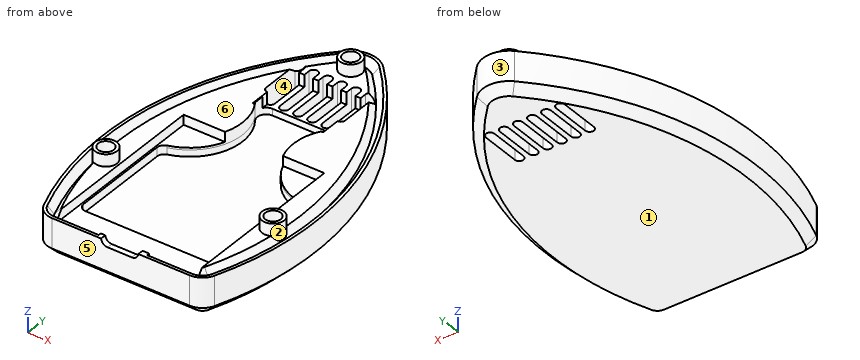
from build123d import *

# Parameters (mm, degrees)
PAD011_DEPTH           = 6.5
CHAMFER_SIZE           = 2
SKETCH020_W            = 32
SKETCH020_H            = 40
POCKET004_DEPTH        = 4.5
SKETCH021_W            = 16
SKETCH021_H            = 13
POCKET005_DEPTH        = 3
POCKET006_DEPTH        = 2
PAD012_DEPTH           = 2.5
POCKET007_DEPTH        = 5
POCKET008_DEPTH        = 6.501
LINEARPATTERN001_COUNT = 6
LINEARPATTERN001_PITCH = 2.8
POCKET009_DEPTH        = 6.501
POCKET009_DEPTH_BACK   = 6.501
LINEARPATTERN002_COUNT = 6
LINEARPATTERN002_PITCH = 3.2
SKETCH043_W            = 50
SKETCH043_H            = 9.25
PAD015_DEPTH           = 80
POCKET010_DEPTH        = 2.751
SKETCH044_R            = 2.5
PAD016_DEPTH           = 5


with BuildPart() as housing:
    # Sketch019 → Pad011 (new body, symmetric)
    with BuildSketch(Plane.XY):
        with BuildLine():
            ThreePointArc((4.279646, 74.20531), (0, 76), (-4.279646, 74.20531))
            ThreePointArc((-4.279646, 74.20531), (-22.568944, 39.95714), (-19.396798, 1.261235))
            ThreePointArc((-19.396798, 1.261235), (-17.9278, -0.59811), (-15.664513, -1.3))
            Line((15.664513, -1.3), (-15.664513, -1.3))
            ThreePointArc((15.664513, -1.3), (17.927792, -0.598116), (19.396791, 1.261217))
            ThreePointArc((19.396791, 1.261217), (22.568946, 39.95713), (4.279646, 74.20531))
        make_face()
    extrude(amount=PAD011_DEPTH, both=True)

    # Chamfer
    chamfer_edges = [housing.edges().sort_by_distance(p)[0] for p in [
        (0, -1.3, 6.5),
        (0, -1.3, -6.5),
    ]]
    chamfer(chamfer_edges, length=CHAMFER_SIZE)

    # Sketch020 → Pocket004 (cut)
    with BuildSketch(Plane.XY):
        with Locations((0, 20)):
            Rectangle(SKETCH020_W, SKETCH020_H)
    extrude(amount=POCKET004_DEPTH, mode=Mode.SUBTRACT)

    # Sketch021 → Pocket005 (cut)
    with BuildSketch(Plane.XY):
        with Locations((0, 57)):
            Rectangle(SKETCH021_W, SKETCH021_H)
    extrude(amount=POCKET005_DEPTH, mode=Mode.SUBTRACT)

    # Sketch022 → Pocket006 (cut, symmetric)
    with BuildSketch(Plane.XY):
        with BuildLine():
            ThreePointArc((-6.35, 54.4), (-8.125922, 53.319838), (-7.98356, 51.246101))
            ThreePointArc((-14.445285, 32.796789), (-6.459474, 40.356063), (-7.98356, 51.246101))
            ThreePointArc((-14.445285, 32.796789), (-15.279151, 32.221131), (-15.6, 31.26))
            Line((-15.6, 8.4), (-15.6, 31.26))
            ThreePointArc((-15.6, 8.4), (-15.131371, 7.268629), (-14, 6.8))
            Line((14, 6.8), (-14, 6.8))
            ThreePointArc((14, 6.8), (15.131371, 7.268629), (15.6, 8.4))
            Line((15.6, 31.26), (15.6, 8.4))
            ThreePointArc((15.6, 31.26), (15.279151, 32.221131), (14.445285, 32.796789))
            ThreePointArc((7.98356, 51.246101), (6.459474, 40.356063), (14.445285, 32.796789))
            ThreePointArc((7.98356, 51.246101), (8.125922, 53.319838), (6.35, 54.4))
            Line((6.35, 54.4), (-6.35, 54.4))
        make_face()
    extrude(amount=POCKET006_DEPTH, both=True, mode=Mode.SUBTRACT)

    # Sketch039 → Pad012 (join)
    with BuildSketch(Plane.XY.offset(-0.5)):
        with BuildLine():
            ThreePointArc((-4.584919, 45.32271), (-5.584919, 44.32271), (-4.584919, 43.32271))
            Line((-4.584919, 43.32271), (4.584919, 43.32271))
            ThreePointArc((4.584919, 43.32271), (5.584919, 44.32271), (4.584919, 45.32271))
            Line((4.584919, 45.32271), (-4.584919, 45.32271))
        make_face()
    extrude(amount=PAD012_DEPTH)

    # Sketch023 → Pocket007 (cut, symmetric)
    with BuildSketch(Plane.XZ):
        with BuildLine():
            ThreePointArc((-3, 3.9), (-4.5, 2.4), (-3, 0.9))
            Line((-3, 0.9), (2.5, 0.9))
            ThreePointArc((2.5, 0.9), (4, 2.4), (2.5, 3.9))
            Line((2.5, 3.9), (-3, 3.9))
        make_face()
    extrude(amount=POCKET007_DEPTH, both=True, mode=Mode.SUBTRACT)

    # Sketch025 → Pocket008 (cut, through all)
    with BuildSketch(Plane.XY):
        with BuildLine():
            ThreePointArc((-6.25, 32.5), (-7, 33.25), (-7.75, 32.5))
            Line((-7.75, 32.5), (-7.75, 13.5))
            ThreePointArc((-7.75, 13.5), (-7, 12.75), (-6.25, 13.5))
            Line((-6.25, 13.5), (-6.25, 32.5))
        make_face()
    pocket008 = extrude(amount=POCKET008_DEPTH, mode=Mode.SUBTRACT)

    # LinearPattern001: Pocket008 ×6
    with Locations(*[(i * LINEARPATTERN001_PITCH, 0, 0) for i in range(1, LINEARPATTERN001_COUNT)]):
        add(pocket008, mode=Mode.SUBTRACT)

    # Sketch026 → Pocket009 (cut, two sides)
    with BuildSketch(Plane.XY) as pocket009_sk:
        with BuildLine():
            ThreePointArc((-7, 65), (-8, 66), (-9, 65))
            Line((-9, 65), (-9, 56))
            ThreePointArc((-9, 56), (-8, 55), (-7, 56))
            Line((-7, 56), (-7, 65))
        make_face()
    pocket009 = extrude(amount=-POCKET009_DEPTH, mode=Mode.SUBTRACT) + extrude(pocket009_sk.sketch, amount=POCKET009_DEPTH_BACK, mode=Mode.SUBTRACT)

    # LinearPattern002: Pocket009 ×6
    with Locations(*[(i * LINEARPATTERN002_PITCH, 0, 0) for i in range(1, LINEARPATTERN002_COUNT)]):
        add(pocket009, mode=Mode.SUBTRACT)

    # Sketch027 → Groove (revolve, cut)
    with BuildSketch(Plane.XZ.offset(-20)):
        Polygon((19, 6.7), (19, -5.8), (19.4, -5.8), (20.8, 5.2), (22.3, 6.7), align=None)
    groove = revolve(axis=Axis((19, 20, 6.7), (0, 0, 1)), mode=Mode.SUBTRACT)

    # Mirrored: Groove across YZ
    add(groove.mirror(Plane.YZ), mode=Mode.SUBTRACT)

    # Sketch028 → Groove001 (revolve, cut)
    with BuildSketch(Plane.XZ.offset(-70)):
        Polygon((0, 6.7), (0, -5.8), (0.4, -5.8), (1.8, 5.2), (3.3, 6.7), align=None)
    revolve(axis=Axis((0, 70, 6.7), (0, 0, 1)), mode=Mode.SUBTRACT)


with BuildPart() as bottom_housing:
    # Sketch043 → Pad015 (new body)
    with BuildSketch(Plane.XZ.offset(2)):
        with Locations((0, -2.375)):
            Rectangle(SKETCH043_W, SKETCH043_H)
    extrude(amount=-PAD015_DEPTH)

    # SubtractivePipe: sweep along a path in Sketch036
    with BuildLine(Plane.XY) as subtractivepipe_path:
        Line((5.5, 0.7), (15.664513, 0.7))
        ThreePointArc((15.664513, 0.7), (16.796157, 1.050945), (17.530656, 1.980617))
        ThreePointArc((17.530656, 1.980617), (20.610558, 39.551278), (2.853097, 72.80354))
        ThreePointArc((2.853097, 72.80354), (0, 74), (-2.853097, 72.80354))
        ThreePointArc((-2.853097, 72.80354), (-20.610558, 39.551278), (-17.530656, 1.980617))
        ThreePointArc((-17.530656, 1.980617), (-16.796157, 1.050945), (-15.664513, 0.7))
        Line((-15.664513, 0.7), (-5.5, 0.7))
    # Sketch037 → SubtractivePipe (sweep, cut)
    with BuildSketch(Plane.YZ):
        Polygon((72.089299, 3), (74, 0.509926), (75.910701, 3), align=None)
    sweep(path=subtractivepipe_path.line, mode=Mode.SUBTRACT)

    # Sketch038 → Pocket010 (cut, through all)
    with BuildSketch(Plane.XY.offset(-0.5)):
        with BuildLine():
            ThreePointArc((7.49701, 50.5), (6.614494, 39.938466), (14.445285, 32.796789))
            Line((14.445285, 32.796789), (-14.445285, 32.796789))
            ThreePointArc((-14.445285, 32.796789), (-6.614494, 39.938466), (-7.49701, 50.5))
            Line((-8, 50.5), (-7.49701, 50.5))
            Line((-8, 63.5), (-8, 50.5))
            Line((8, 63.5), (-8, 63.5))
            Line((8, 50.5), (8, 63.5))
            Line((7.49701, 50.5), (8, 50.5))
        make_face()
    extrude(amount=POCKET010_DEPTH, mode=Mode.SUBTRACT)

    # Sketch044 → Pad016 (join)
    with BuildSketch(Plane.XY):
        with Locations((0, 70)):
            Circle(SKETCH044_R)
        with Locations((-19, 20)):
            Circle(SKETCH044_R)
        with Locations((19, 20)):
            Circle(SKETCH044_R)
    extrude(amount=PAD016_DEPTH)

    # Common001: intersect Housing
    add(housing.part, mode=Mode.INTERSECT)


solid = bottom_housing.part
Read the model definition and answer for the solid it produces. Units are mm, in the model's axes. Face numbers are marked on the shaded views. A direction names the side the tool comes from. Coordinates: 2 decimals unless noted, no trailing zeros. Write each loop counter-clockwise with the first axis right and the second up, starting at its lowest first coordinate (ties: lowest second). Pieces come first, ordered by that corner, then holes. Notation, with made-up numbers: (-31.75, 42.25) -> (19.25, 42.25) arc R34 ccw to (19.25, 74.25) -> close; hole circle Ø2 at (9, 81.25). An arc over 180 degrees is marked (long way). Return JSON: item names as keys, results as strings.
(1) The part is cut by section B-B on z = -3.75. State how many separate pieces and enclosed holes the cut face has, then the cut area to 3 significant figures.
Answers below:
{"separate pieces": "1", "enclosed holes": "9", "area": "2,810 mm^2"}
(2) Consider line 1 along X through (y, z) = (21, 1.5); line 2 along X through (y, z) = (44.5, 1.75); line 3 along X through (y, z) = (18.5, 1). Determine where each line is inside the solid, lowest interval first. Write a range as from..to.
Answers below:
{"line 1": "-23.82..-22.57, -21.29..-19.88, -18.12..-16, 16..18.12, 19.88..21.29, 22.57..23.82", "line 2": "-21.47..-20.38, -18.4..-5.79, 5.79..18.4, 20.38..21.47", "line 3": "-23.59..-21.96, -21.2..-16, 16..21.2, 21.96..23.59"}
(3) The part is cut by section A-A on z = 3.5. Give the vertices of the cut face in (x, y), then the cut area to 3 significant figures.
Answers below:
{"outline": "circle Ø5 at (-19, 20); circle Ø5 at (0, 70); circle Ø5 at (19, 20); hole circle Ø3.17 at (-19, 20); hole circle Ø3.17 at (0, 70); hole circle Ø3.17 at (19, 20)", "area": "35.3 mm^2"}
(4) Which of the six approach directions +Z, -Z, +X, -X, +Y, -Y give full straight-line access (tool end or side, diameter ignored) to the marked faces 1 and 2?
Answers below:
{"face 1": "-Z, +X, -X, +Y, -Y", "face 2": "+Z"}
(5) Each of these flat-tipped pins is pushed along its axis until it touches: P1, Ø8, axis at x = 1, y = 59, coming from the +Z side; P2, Ø1.1, axis at y = 17.5, z = 0.5, coming from the +X side; P3, Ø2, axis at y = 8, z = -4.5, coming from the +X side. Where does it stop, or does it pass through?
Answers below:
{"P1": "z = -0.5", "P2": "x = 23.54", "P3": "x = 21.87"}
(6) For a pull along Y with two mould halves and no side action, classify the marked faces 3, 4, 5 and 6 as pulls with the +Y half, pulls with the -Y half, needs draft (parallel to the pull), parting line crosses it, or undercut.
Answers below:
{"face 3": "pulls with the +Y half", "face 4": "undercut", "face 5": "pulls with the -Y half", "face 6": "needs draft"}
